```python
from build123d import *

# Parameters (mm, degrees)
F0_R     = 6
F1_DEPTH = 15
F2_DEPTH = 15
F0_R_2   = 2.36
F3_DEPTH = 11
F5_DEPTH = 25
F6_DEPTH = 3.4


with BuildPart() as f1:
    # F0 (on Front) → F1 (new body)
    with BuildSketch(Plane.XZ):
        with BuildLine():
            ThreePointArc((7.834258, -1.62), (7.958457, -0.814228), (8, 0))
            ThreePointArc((8, 0), (7.958457, 0.814228), (7.834258, 1.62))
            ThreePointArc((7.834258, 1.62), (5.678687, 5.634937), (1.680542, 7.821495))
            ThreePointArc((1.680542, 7.821495), (-8, 0), (1.680542, -7.821495))
            ThreePointArc((1.680542, -7.821495), (5.678687, -5.634937), (7.834258, -1.62))
        make_face()
        Circle(F0_R, mode=Mode.SUBTRACT)
    extrude(amount=F1_DEPTH)

    # F0 (on Front) → F2 (join)
    with BuildSketch(Plane.XZ):
        with BuildLine():
            ThreePointArc((7.834258, 1.62), (7.958457, 0.814228), (8, 0))
            ThreePointArc((8, 0), (7.958457, -0.814228), (7.834258, -1.62))
            Line((7.834258, -1.62), (17.378049, -1.62))
            ThreePointArc((17.378049, -1.62), (17, 0), (17.378049, 1.62))
            Line((17.378049, 1.62), (7.834258, 1.62))
        make_face()
    extrude(amount=F2_DEPTH)

    # F0 (on Front) → F3 (join)
    with BuildSketch(Plane.XZ):
        with BuildLine():
            ThreePointArc((21.428848, 3.578334), (19.066987, 3.295134), (17.378049, 1.62))
            ThreePointArc((17.378049, 1.62), (17, 0), (17.378049, -1.62))
            ThreePointArc((17.378049, -1.62), (19.066987, -3.295134), (21.428848, -3.578334))
            ThreePointArc((21.428848, -3.578334), (23.506892, -2.300176), (24.32, 0))
            ThreePointArc((24.32, 0), (23.506892, 2.300176), (21.428848, 3.578334))
        make_face()
        with Locations((20.66, 0)):
            Circle(F0_R_2, mode=Mode.SUBTRACT)
    extrude(amount=F3_DEPTH)

    # F4 (on face) → F5 (cut)
    with BuildSketch(Plane(origin=(0, 0, -1.62), x_dir=(1, 0, 0), z_dir=(0, 0, -1))):
        Polygon((17.378049, 15), (7.834258, 15), (17.378049, 11), align=None)
    extrude(amount=-F5_DEPTH, mode=Mode.SUBTRACT)

    # F0 (on Front) → F6 (join)
    with BuildSketch(Plane.XZ):
        with BuildLine():
            ThreePointArc((1.680542, 7.821495), (5.678687, 5.634937), (7.834258, 1.62))
            Line((7.834258, 1.62), (17.378049, 1.62))
            ThreePointArc((17.378049, 1.62), (19.066987, 3.295134), (21.428848, 3.578334))
            Line((21.428848, 3.578334), (1.680542, 7.821495))
        make_face()
        with BuildLine():
            Line((17.378049, -1.62), (7.834258, -1.62))
            ThreePointArc((7.834258, -1.62), (5.678687, -5.634937), (1.680542, -7.821495))
            Line((1.680542, -7.821495), (21.428848, -3.578334))
            ThreePointArc((21.428848, -3.578334), (19.066987, -3.295134), (17.378049, -1.62))
        make_face()
    extrude(amount=F6_DEPTH)


solid = f1.part
```
Check sheet for the modelled part. Datum: model origin and axes. Units: mm. A direction names the side the tool comes from. Coordinates: 2 decimals unless noted, no trailing zeros. Write each loop counter-clockwise with the first axis right and the second up, starting at its lowest first coordinate (ties: lowest second). Pieces come first, ordered by that corner, then holes. Notation, with made-up numbers: M -1.5,55 L 28.5,55 A21 cw 28.5,86 Z; hole C 74,85 d1. An arc over 180 degrees is marked long. Write item = value, one per line. Start each with the question number.
1. Go/stop test with flat-tipped pins: pin 1 (7.5 mm diameter, centred on x = 12.5, y = -8, fed in from +Z); pin 2 (5 mm diameter, centred on x = 13.5, z = 4, fed in from -Y); pin 3 (2 mm diameter, centred on y = -12.5, z = 5.5, fed in from +X). Record where each tip stops, or that it passes through.
2. Thickness scan on probe 1 along Z at (x, y) = (20.5, -6.5); probe 2 along Z at (x, y) = (0, -10); probe 3 along X at (y, z) = (-7, -1.5). Record the ranges inside material, lowest first.
3. Sectioned sample at D-D (y = -11.75). Record the cut outline in (x, z).
4. Sectioned sample at B-B (y = -2.75). Record the cut outline in (x, z), then the cut area to 3 significant figures.
5. Sectioned sample at C-C (z = 1). Record the cut outline in (x, y).
6. Mould release check, pull along X, two halves, no side actions. Record for faces 4 (the flat face through (11, -3.4, -4)), 5 (the flat face through (11.69, -1.68, 5.67)), 6 (the flat face through (8, 0, 0)), 7 (the flat face through (13, -8, 1.62)): pulls with the +X half, pulls with the -X half, needs draft (parallel to the pull), parting line crosses it, or undercut.
7. Tool access check on faces 1 (the flat face through (11, -3.4, 4)), 2 (the flat face through (12.539, -13.028, -0.023)), 3 (the flat face through (13, -8, -1.62)). Record the directions out of +Z, -Z, +X, -X, +Y, -Y that give a thin tool (end or side, any length) a straight path to the whole face; none if there is none.
8. Sectioned sample at A-A (x = 0). Record the cut outline in (y, z), then the cut area to 3 significant figures.
The answers:
q1.pin_1 = 1.62
q1.pin_2 = -12.95
q1.pin_3 = 6.61
q2.probe_1 = -3.66 to -2.35, 2.35 to 3.66
q2.probe_2 = -8 to -6, 6 to 8
q2.probe_3 = -7.86 to -5.81, 5.81 to 18.84, 22.48 to 24
q3.outline = M 7.83,-1.62 L 15.59,-1.62 L 15.59,1.62 L 7.83,1.62 A8 ccw long Z; hole C 0,0 d12
q4.outline = M 1.68,-7.82 L 21.43,-3.58 A3.66 ccw 24.32,0 A3.66 ccw 21.43,3.58 L 1.68,7.82 A8 ccw long Z; hole C 0,0 d12; hole C 20.66,0 d4.72
q4.area = 237 mm²
q5.outline = M -7.94,-15 L -5.92,-15 L -5.92,0 L -7.94,0 Z; M 5.92,-15 L 7.83,-15 L 17.14,-11.1 L 17.14,-11 L 18.52,-11 L 18.52,0 L 5.92,0 Z; M 22.8,-11 L 24.18,-11 L 24.18,0 L 22.8,0 Z
q6.face_4 = undercut
q6.face_5 = pulls with the +X half
q6.face_6 = needs draft
q6.face_7 = undercut
q7.face_1 = +Z, -Y
q7.face_2 = +Z, -Z, +X, -Y
q7.face_3 = -Z, -Y
q8.outline = M -15,-8 L 0,-8 L 0,-6 L -15,-6 Z; M -15,6 L 0,6 L 0,8 L -15,8 Z
q8.area = 60.0 mm²
